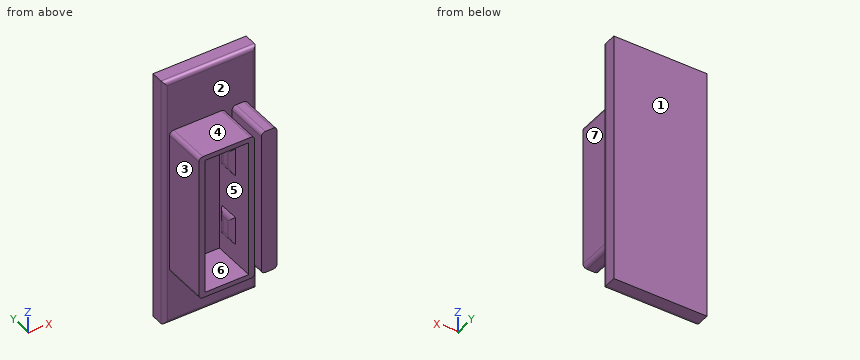
from build123d import *

# Parameters (mm, degrees)
F0_W        = 10.795
F0_H        = 25.4
F1_DEPTH    = 2.54
F2_W        = 8.89
F2_H        = 23.495
F2_W_2      = 6.985
F2_H_2      = 21.971
F3_DEPTH    = 6.985
F4_W        = 3.175
F4_H        = 4.445
F5_DEPTH    = 0.5
F6_W        = 3.175
F6_H        = 4.445
F7_DEPTH    = 0.5
F8_T1_DEPTH = 5.6998762346
F8_T3_DEPTH = 9.4947524692
F8_T5_DEPTH = 9.4947524692
F9_W        = 10.795
F9_H        = 7.5
F10_DEPTH   = 2.54
F11_W       = 2.5
F11_H       = 23.495
F12_DEPTH   = 6.985
F13_R       = 0.635


# Not quite as in the source:
# - a fillet or chamfer that OpenCascade refuses, or shapes differently, is made with other operations: its cross-section is extruded or revolved along the edge and cut away or added


with BuildPart() as f1:
    # F0 (on Front) → F1 (new body)
    with BuildSketch(Plane.XZ):
        with Locations((5.3975, -12.7)):
            Rectangle(F0_W, F0_H)
    extrude(amount=F1_DEPTH)

    # F2 (on face) → F3 (join)
    with BuildSketch(Plane.XZ.offset(2.54)):
        with Locations((5.3975, -12.7)):
            Rectangle(F2_W, F2_H)
        with Locations((5.3975, -12.7)):
            Rectangle(F2_W_2, F2_H_2, mode=Mode.SUBTRACT)
    extrude(amount=F3_DEPTH)

    # F4 (on face) → F5 (join)
    with BuildSketch(Plane.YZ.offset(1.905)):
        with Locations((-4.7625, -6.985)):
            Rectangle(F4_W, F4_H)
        with Locations((-4.7625, -18.415)):
            Rectangle(F4_W, F4_H)
    extrude(amount=F5_DEPTH)

    # F6 (on face) → F7 (join)
    with BuildSketch(Plane(origin=(8.89, 0, 0), x_dir=(0, -1, 0), z_dir=(-1, 0, 0))):
        with Locations((4.7625, -6.985)):
            Rectangle(F6_W, F6_H)
        with Locations((4.7625, -18.415)):
            Rectangle(F6_W, F6_H)
    extrude(amount=F7_DEPTH)

    # F8: fillet of radius 1.27 on 16 edges, made by hand

    # F8_s2 → F8_t1 (cut)
    with BuildSketch(Plane.XZ.offset(3.175)):
        with BuildLine():
            ThreePointArc((1.905, -16.1925), (2.273156404, -16.6389791104), (2.405, -17.2024504938))
            Line((2.405, -17.2024504938), (2.405, -16.1925))
            Line((2.405, -16.1925), (1.905, -16.1925))
        make_face()
        with BuildLine():
            ThreePointArc((1.905, -20.6375), (2.273156404, -20.1910208896), (2.405, -19.6275495062))
            Line((2.405, -19.6275495062), (2.405, -20.6375))
            Line((2.405, -20.6375), (1.905, -20.6375))
        make_face()
        with BuildLine():
            ThreePointArc((1.905, -4.7625), (2.273156404, -5.2089791104), (2.405, -5.7724504938))
            Line((2.405, -5.7724504938), (2.405, -4.7625))
            Line((2.405, -4.7625), (1.905, -4.7625))
        make_face()
        with BuildLine():
            ThreePointArc((1.905, -9.2075), (2.273156404, -8.7610208896), (2.405, -8.1975495062))
            Line((2.405, -8.1975495062), (2.405, -9.2075))
            Line((2.405, -9.2075), (1.905, -9.2075))
        make_face()
        with BuildLine():
            ThreePointArc((8.89, -4.7625), (8.521843596, -5.2089791104), (8.39, -5.7724504938))
            Line((8.39, -5.7724504938), (8.39, -4.7625))
            Line((8.39, -4.7625), (8.89, -4.7625))
        make_face()
        with BuildLine():
            ThreePointArc((8.89, -9.2075), (8.521843596, -8.7610208896), (8.39, -8.1975495062))
            Line((8.39, -8.1975495062), (8.39, -9.2075))
            Line((8.39, -9.2075), (8.89, -9.2075))
        make_face()
        with BuildLine():
            ThreePointArc((8.89, -16.1925), (8.521843596, -16.6389791104), (8.39, -17.2024504938))
            Line((8.39, -17.2024504938), (8.39, -16.1925))
            Line((8.39, -16.1925), (8.89, -16.1925))
        make_face()
        with BuildLine():
            ThreePointArc((8.89, -20.6375), (8.521843596, -20.1910208896), (8.39, -19.6275495062))
            Line((8.39, -19.6275495062), (8.39, -20.6375))
            Line((8.39, -20.6375), (8.89, -20.6375))
        make_face()
    extrude(amount=F8_T1_DEPTH, mode=Mode.SUBTRACT)

    # F8_s4 → F8_t3 (cut)
    with BuildSketch(Plane.XY.offset(-23.1623762346)):
        with BuildLine():
            ThreePointArc((1.905, -6.35), (2.273156404, -5.9035208896), (2.405, -5.3400495062))
            Line((2.405, -5.3400495062), (2.405, -6.35))
            Line((2.405, -6.35), (1.905, -6.35))
        make_face()
        with BuildLine():
            ThreePointArc((1.905, -3.175), (2.273156404, -3.6214791104), (2.405, -4.1849504938))
            Line((2.405, -4.1849504938), (2.405, -3.175))
            Line((2.405, -3.175), (1.905, -3.175))
        make_face()
        with BuildLine():
            ThreePointArc((8.89, -3.175), (8.521843596, -3.6214791104), (8.39, -4.1849504938))
            Line((8.39, -4.1849504938), (8.39, -3.175))
            Line((8.39, -3.175), (8.89, -3.175))
        make_face()
        with BuildLine():
            ThreePointArc((8.89, -6.35), (8.521843596, -5.9035208896), (8.39, -5.3400495062))
            Line((8.39, -5.3400495062), (8.39, -6.35))
            Line((8.39, -6.35), (8.89, -6.35))
        make_face()
    extrude(amount=F8_T3_DEPTH, mode=Mode.SUBTRACT)

    # F8_s6 → F8_t5 (cut)
    with BuildSketch(Plane.XY.offset(-11.7323762346)):
        with BuildLine():
            ThreePointArc((1.905, -6.35), (2.273156404, -5.9035208896), (2.405, -5.3400495062))
            Line((2.405, -5.3400495062), (2.405, -6.35))
            Line((2.405, -6.35), (1.905, -6.35))
        make_face()
        with BuildLine():
            ThreePointArc((1.905, -3.175), (2.273156404, -3.6214791104), (2.405, -4.1849504938))
            Line((2.405, -4.1849504938), (2.405, -3.175))
            Line((2.405, -3.175), (1.905, -3.175))
        make_face()
        with BuildLine():
            ThreePointArc((8.89, -3.175), (8.521843596, -3.6214791104), (8.39, -4.1849504938))
            Line((8.39, -4.1849504938), (8.39, -3.175))
            Line((8.39, -3.175), (8.89, -3.175))
        make_face()
        with BuildLine():
            ThreePointArc((8.89, -6.35), (8.521843596, -5.9035208896), (8.39, -5.3400495062))
            Line((8.39, -5.3400495062), (8.39, -6.35))
            Line((8.39, -6.35), (8.89, -6.35))
        make_face()
    extrude(amount=F8_T5_DEPTH, mode=Mode.SUBTRACT)

    # F9 (on Front) → F10 (join)
    with BuildSketch(Plane.XZ):
        with Locations((5.3975, 3.75)):
            Rectangle(F9_W, F9_H)
        Polygon((10.795, 7.5), (10.795, 0), (10.795, -25.4), (10.795, -32.9), (14.8425, -32.9), (14.8425, 7.5), align=None)
        with Locations((5.3975, -29.15)):
            Rectangle(F9_W, F9_H)
    extrude(amount=F10_DEPTH)

    # F11 (on face) → F12 (join)
    with BuildSketch(Plane.XZ.offset(2.54)):
        with Locations((12.1425, -12.7)):
            Rectangle(F11_W, F11_H)
    extrude(amount=F12_DEPTH)

    # F13
    f13_edges = [f1.edges().sort_by_distance(p)[0] for p in [
        (0.9525, -6.0325, -0.9525),
        (9.8425, -6.0325, -0.9525),
        (9.8425, -6.0325, -24.4475),
        (0.9525, -6.0325, -24.4475),
        (0, -2.54, -12.7),
        (10.8925, -6.0325, -24.4475),
        (13.3925, -6.0325, -24.4475),
        (10.8925, -6.0325, -0.9525),
        (13.3925, -6.0325, -0.9525),
        (14.8425, -2.54, -12.7),
        (7.42125, -2.54, -32.9),
        (7.42125, -2.54, 7.5),
    ]]
    fillet(f13_edges, radius=F13_R)


solid = f1.part
The model under review builds one solid part; all positions refer to its coordinate system, in mm. Face numbers are marked on the shaded views. A direction names the side the tool comes from. Round coordinates to 2 decimals unless told otherwise and drop trailing zeros. Loops run counter-clockwise (first coordinate to the right, second up) from the corner with the lowest first, then second, coordinate; pieces in that order, holes last. Notation, with made-up numbers: (-22, -27.5) -> (9, -27.5) arc R21 cw to (9, -5.5) -> close; hole circle Ø5 at (-10.5, 72.25). An arc over 180 degrees is marked (long way). One line per question, with ' | ' between items. Start each with the question number.
Item 1: Wall thickness on line 1 along X through (y, z) = (-4.25, -18.5) (1 decimal); line 2 along X through (y, z) = (-7.25, -13.5) (1 decimal); line 3 along Z through (x, y) = (6.5, -6.5): over which ranges is each line inside the solid? List them lowest first. Write a range as [from, to].
Item 2: Add section A-A, the plane y = -8.5. Write out the cut boundary in (x, z) (1 decimal).
Item 3: Draft analysis for pull direction Z (two halves, no side actions). For the marked faces 4, 5, 6 and 7, state which applies: +Z half, -Z half, draft (parallel to the pull), parting line (faces both ways), or undercut.
Item 4: Add section D-D, the plane z = -29. Write out the cut boundary in (x, y) (1 decimal).
Item 5: Machinability: for the marked faces 1, 2 and 3, which of the approach directions +Z, -Z, +X, -X, +Y, -Y give a long, thin tool a straight path to every point of the face, cutting with its end or side? Answer none if there is none.
Item 6: Add section C-C, the plane x = 7. Write out the cut boundary in (y, z) (1 decimal).
Item 7: For pin 1 (3 mm diameter, centred on x = 13, z = -22.5, fed in from +Y); pin 2 (5.5 mm diameter, centred on y = -7.5, z = -16, fed in from +X); pin 3 (4 mm diameter, centred on y = -5, z = -22, fed in from -X); pin 4 (2 mm diameter, centred on x = 7, z = -12.5, fed in from -Y), all flat-tipped, find the tip position at first contact; note any pin that passes through.
Return value:
1) line 1: x = [1, 2.4], [8.4, 9.8], [10.9, 13.4] | line 2: x = [1, 1.9], [8.9, 9.8], [10.9, 13.4] | line 3: z = [-24.45, -23.69], [-1.71, -0.95]
2) outline: (1, -23.8) arc R0.6 ccw to (1.6, -24.4) -> (9.2, -24.4) arc R0.6 ccw to (9.8, -23.8) -> (9.8, -1.6) arc R0.6 ccw to (9.2, -1) -> (1.6, -1) arc R0.6 ccw to (1, -1.6) -> close; (10.9, -23.8) arc R0.6 ccw to (11.5, -24.4) -> (12.8, -24.4) arc R0.6 ccw to (13.4, -23.8) -> (13.4, -1.6) arc R0.6 ccw to (12.8, -1) -> (11.5, -1) arc R0.6 ccw to (10.9, -1.6) -> close; hole (1.9, -23.7) -> (8.9, -23.7) -> (8.9, -1.7) -> (1.9, -1.7) -> close
3) face 4: +Z half | face 5: undercut | face 6: undercut | face 7: draft
4) outline: (0, -1.9) arc R0.6 ccw to (0.6, -2.5) -> (14.2, -2.5) arc R0.6 ccw to (14.8, -1.9) -> (14.8, 0) -> (0, 0) -> close
5) face 1: +Z, -Z, +X, -X, +Y | face 2: -Y | face 3: +Z, -Z, -X, -Y
6) outline: (-9.5, -24.4) -> (-2.5, -24.4) -> (-2.5, -32.3) arc R0.6 ccw to (-1.9, -32.9) -> (0, -32.9) -> (0, 7.5) -> (-1.9, 7.5) arc R0.6 ccw to (-2.5, 6.9) -> (-2.5, -1) -> (-9.5, -1) -> (-9.5, -1.7) -> (-2.5, -1.7) -> (-2.5, -23.7) -> (-9.5, -23.7) -> close
7) pin 1: stops at y = 0 | pin 2: stops at x = 13.39 | pin 3: stops at x = 0.95 | pin 4: stops at y = -2.54
